The listing builds one solid part. Answer for the finished solid, in the listing's coordinates (mm). A direction names the side the tool comes from. Give positions to 0.01 mm unless a question says otherwise; leave off trailing zeros. Order: outer loops, then holes, each group sorted by start corner. A loop starts at its lowest first (then second) coordinate and runs counter-clockwise, first axis right, second up. Notation, with made-up numbers: (16.25, 74) - (49.25, 74) arc R33 ccw to (49.25, 107) - close; hole circle Ø4 at (-3.75, -5). An arc over 180 degrees is marked (long way). Use a Markdown table: item, result. Add a question column.
1) Find section B-B, the plane y = 21.5. State how many separate pieces and enclosed holes the cut face has, plus the area to 3 significant figures.
2) Find section C-C, the plane z = -101. Determine the outline of the cut face in (x, y).
3) For faces 1 (the face through (231.19, 12.88, 86.07)), 2 (the face through (123, 0, 2)), determine the directions among +Z, -Z, +X, -X, +Y, -Y from which every point of the face is accessible in a straight line to the end or side of a thin tool.
4) The mould has two halves that part along Z. Classify faces 3 (the face through (123, 13, 152.4)), 4 (the face through (123, 25.4, 2)), 5 (the face through (166.48, 12.52, -119.67)), 6 (the face through (123, 13, -152.4)): released by +Z, released by -Z, zero draft, split by the parting line, or undercut.
5) Find section A-A, the plane x = 355.6. Determine the outline of the cut face in (y, z) (3 decimals).
6) A flat-ended cylindrical pin translates along its axis: pin 1 (19 mm diameter, centred on x = 152.4, z = 127, fed in from -Y). Find the tip coordinate at first contact, or state that the pin passes through.
7) Straight lines are drawn through the part: line 1 (Z direction, x = 355.6, y = 6) (3 decimals); line 2 (X direction, y = 15.75, z = -127) (3 decimals); line 3 (Z direction, x = 7.5, y = 16.5). For each, find the intervals that lie inside material, in ascending order.
from build123d import *

# Parameters (mm, degrees)
SKETCH1_W           = 127
SKETCH1_H           = 152.4
SKETCH1_R           = 15.875
BOSS_EXTRUDE1_DEPTH = 25.4
CUT_EXTRUDE1_DEPTH  = 25.4


with BuildPart() as part:
    # Sketch1 → Boss-Extrude1 (new body)
    with BuildSketch(Plane(origin=(0, 0, 0), x_dir=(1, 0, 0), z_dir=(0, 1, 0))):
        with Locations((63.5, 76.2)):
            Rectangle(SKETCH1_W, SKETCH1_H)
        with Locations(Location((101.6, 127, 0), (0, 0, 270))):
            Circle(SKETCH1_R, mode=Mode.SUBTRACT)
    boss_extrude1 = extrude(amount=BOSS_EXTRUDE1_DEPTH)

    # Mirror1: Boss-Extrude1 across plane
    add(boss_extrude1.mirror(Plane(origin=(0, 25.4, 0), x_dir=(1, 0, 0), z_dir=(0, 0, -1))))

    # Mirror2: part across plane


with BuildPart() as part_1:
    add(part.part)
    add(part.part.mirror(Plane(origin=(0, 25.4, -152.4), x_dir=(0, 0, 1), z_dir=(1, 0, 0))))

    # Sketch2 → Cut-Extrude1 (cut)
    with BuildSketch(Plane(origin=(0, 25.4, 0), x_dir=(1, 0, 0), z_dir=(0, 1, 0))):
        Polygon((44.642701317, 47.647498522), (0.35523126, 125.58620398), (-44.997932577, 48.262777112), align=None)
    cut_extrude1 = extrude(amount=-CUT_EXTRUDE1_DEPTH, mode=Mode.SUBTRACT)

    # Mirror3: Cut-Extrude1 across plane
    add(cut_extrude1.mirror(Plane.XY), mode=Mode.SUBTRACT)

    # Mirror4: part across plane


with BuildPart() as part_2:
    add(part_1.part)
    add(part_1.part.mirror(Plane(origin=(127, 25.4, -152.4), x_dir=(0, 0, 1), z_dir=(-1, 0, 0))))


solid = part_2.part
The answers:
| question | item | result |
|---|---|---|
| 1 | separate pieces | 1 |
| 1 | enclosed holes | 12 |
| 1 | area | 135,000 mm2 |
| 2 | outline | (-127, 0) - (-14.07, 0) - (-14.07, 25.4) - (-127, 25.4) - close; (14.33, 0) - (239.67, 0) - (239.67, 25.4) - (14.33, 25.4) - close; (268.07, 0) - (381, 0) - (381, 25.4) - (268.07, 25.4) - close |
| 3 | face 1 | +Y, -Y |
| 3 | face 2 | +Z, -Z, +X, -X, -Y |
| 4 | face 3 | released by +Z |
| 4 | face 4 | zero draft |
| 4 | face 5 | undercut |
| 4 | face 6 | released by -Z |
| 5 | outline | (0, -152.4) - (25.4, -152.4) - (25.4, -142.875) - (0, -142.875) - close; (0, -111.125) - (25.4, -111.125) - (25.4, 111.125) - (0, 111.125) - close; (0, 142.875) - (25.4, 142.875) - (25.4, 152.4) - (0, 152.4) - close |
| 6 | pin 1 | through |
| 7 | line 1 | -152.4 to -142.875, -111.125 to 111.125, 142.875 to 152.4 |
| 7 | line 2 | -127 to -117.475, -85.725 to 85.725, 117.475 to 136.525, 168.275 to 339.725, 371.475 to 381 |
| 7 | line 3 | -152.4 to -113.01, -47.9 to 47.9, 113.01 to 152.4 |
